Could you check a few things on this drawing? It's one solid part, dimensions in mm from its lowest x, y, z. Coordinates: 2 decimals unless noted, no trailing zeros. Write each loop counter-clockwise with the first axis right and the second up, starting at its lowest first coordinate (ties: lowest second). Pieces come first, ordered by that corner, then holes.
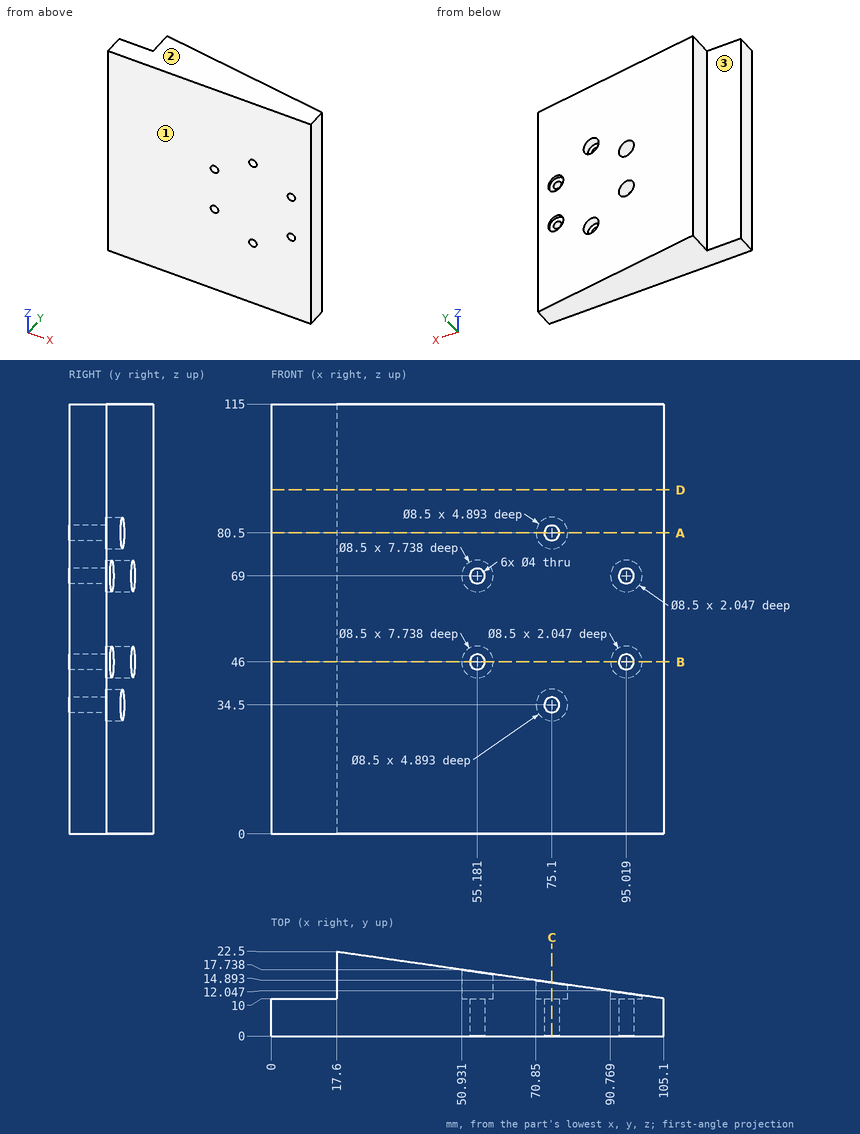
1) Imagine slicing it at D-D on z = 92. Please give me the cut outline in (x, y), then the cut area to 3 significant figures.
Values follow:
outline: (0, 0) - (105.1, 0) - (105.1, 10) - (17.6, 22.5) - (17.6, 10) - (0, 10) - close
area: 1,600 mm2
2) I need wall thicknesses on probe 1 along Z at (x, y) = (75, 3.25); probe 2 along Z at (x, y) = (75.1, 12.4); probe 3 along X at (y, z) = (2.5, 34.5). Which ranges of each line are inside material? Lowest first, please.
Values follow:
probe 1: z = 0 to 32.5, 36.5 to 78.5, 82.5 to 115
probe 2: z = 0 to 30.25, 38.75 to 76.25, 84.75 to 115
probe 3: x = 0 to 73.1, 77.1 to 105.1
3) Imagine slicing it at A-A on z = 80.5. Please give me the cut outline in (x, y).
Values follow:
outline: (0, 0) - (73.1, 0) - (73.1, 10) - (70.85, 10) - (70.85, 14.89) - (17.6, 22.5) - (17.6, 10) - (0, 10) - close; (77.1, 0) - (105.1, 0) - (105.1, 10) - (79.35, 13.68) - (79.35, 10) - (77.1, 10) - close
4) Will these pins go through, and if not, where does the flat tip stop? pin 1 (1.5 mm diameter, centred on x = 29.5, z = 64.5, fed in from -Y); pin 2 (3.5 mm diameter, centred on x = 75.1, z = 34.5, fed in from -Y); pin 3 (9.5 mm diameter, centred on x = 73.5, z = 34.5, fed in from +Y); pin 4 (6.5 mm diameter, centred on x = 55.18, z = 69, fed in from +Y).
Values follow:
pin 1: stops at y = 0
pin 2: passes through
pin 3: stops at y = 15.19
pin 4: stops at y = 10
5) Imagine slicing it at C-C on x = 75.1. Count the separate pieces of the cut face and the enclosed holes in it, then the cut area to 3 significant figures.
Values follow:
separate pieces: 3
enclosed holes: 0
area: 1,490 mm2
6) We'd pull the mould along Y, two halves only. Please class the marked faces 1, 2 and 3: pulls with the +Y half, pulls with the -Y half, needs draft (parallel to the pull), parting line crosses it, or undercut.
Values follow:
face 1: pulls with the -Y half
face 2: needs draft
face 3: pulls with the +Y half
7) Imagine slicing it at B-B on z = 46. Please give me the cut outline in (x, y), then the cut area to 4 significant figures.
Values follow:
outline: (0, 0) - (53.18, 0) - (53.18, 10) - (50.93, 10) - (50.93, 17.74) - (17.6, 22.5) - (17.6, 10) - (0, 10) - close; (57.18, 0) - (93.02, 0) - (93.02, 10) - (90.77, 10) - (90.77, 12.05) - (59.43, 16.52) - (59.43, 10) - (57.18, 10) - close; (97.02, 0) - (105.1, 0) - (105.1, 10) - (99.27, 10.83) - (99.27, 10) - (97.02, 10) - close
area: 1,445 mm2
